The listing builds one solid part. Answer for the finished solid, in the listing's coordinates (mm). Face numbers are marked on the shaded views. Give positions to 0.01 mm unless a question says otherwise; leave off trailing zeros. Write each loop counter-clockwise with the first axis right and the second up, starting at its lowest first coordinate (ties: lowest second). Pieces come first, ordered by that corner, then holes. Notation, with made-up numbers: (55.25, 7.25) - (91.25, 7.25) arc R19 cw to (91.25, 38.25) - close; hole circle Ø3 at (34, -14.5). An arc over 180 degrees is marked (long way). One line per question, with ' | ' between items. Start each with the question number.
1. Find the intervals of material crossed by L1, parallel to X at y = -0.45, z = -81; L2, parallel to X at y = 0.5, z = -32.5; L3, parallel to Z at x = -5, y = 0.4, in increasing order. Write a range as from..to.
2. A cutting plane is placed at C-C (x = -2). Determine the outline of the cut face in (y, z), then the cut area to 4 significant figures.
3. A cutting plane is placed at A-A (z = -71.5). Determine the outline of the cut face in (x, y).
4. The mould has two halves that part along Z. Classify the marked faces 1 and 2: +Z half, -Z half, draft (parallel to the pull), parting line (faces both ways), or undercut.
5. A cutting plane is placed at B-B (y = -1.6). Determine the outline of the cut face in (x, z).
6. A cutting plane is placed at D-D (z = -42). Determine the outline of the cut face in (x, y), then the cut area to 4 significant figures.
7. Given P1, Ø3, axis at x = -39, z = -6.5, coming from the +Y side; P2, Ø3, axis at x = -36.5, y = -2, coming from the -Z side, each flat-ended and moving along its own axis, determine where each tip first touches the part or whether it passes through.
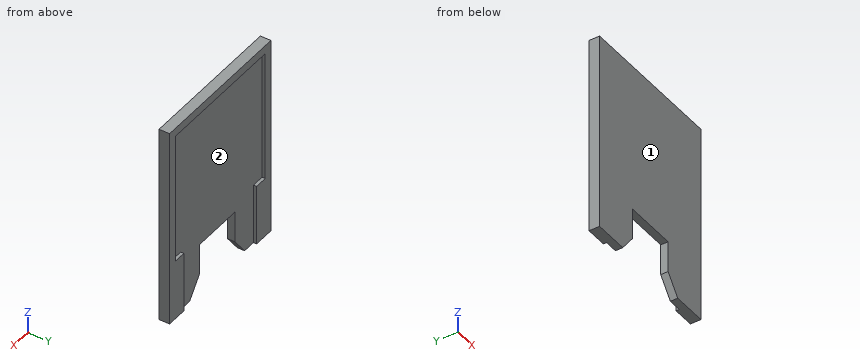
Autodesk Inventor part; units mm, degrees
ref_plane "YZ Plane" through (0, 0, 0) normal (1, 0, 0) x (0, 1, 0)
ref_plane "XZ Plane" through (0, 0, 0) normal (0, 1, 0) x (-1, 0, 0)
ref_plane "XY Plane" through (0, 0, 0) normal (0, 0, 1) x (1, 0, 0)
sketch "Skizze1" plane through (0, 0, 0) normal (0, 1, 0) x (-1, 0, 0)
  line L0 (0, 0) -> (63, 0)
  line L1 (63, 0) -> (63, -63)
  line L2 (63, -63) -> (0, -63)
  line L3 (0, -63) -> (0, 0)
  line L4 (-4, 4) -> (67, 4)
  line L5 (67, 4) -> (67, -92)
  line L6 (67, -92) -> (-4, -92)
  line L7 (-4, -92) -> (-4, 4)
  line L8 (57, -63) -> (6, -63)
  line L9 (6, -63) -> (6, -68)
  line L10 (6, -68) -> (57, -68)
  line L11 (57, -68) -> (57, -63)
  line L12 (44, -68) -> (19, -68)
  line L13 (19, -68) -> (19, -92)
  line L14 (19, -92) -> (44, -92)
  line L15 (44, -92) -> (44, -68)
  line L16 (44, -68) -> (44, -83)
  line L17 (44, -83) -> (44, -93)
  line L18 (44, -93) -> (49.7342, -93)
  line L19 (49.7342, -93) -> (44, -83)
  line L20 (49.1608, -92) -> (44, -92)
  line L21 (19, -83) -> (19, -93)
  line L22 (19, -93) -> (11.5, -93)
  line L23 (11.5, -93) -> (19, -83)
  line L24 (12.25, -92) -> (19, -92)
  line L25 (57, -68) -> (57, -71.1865)
  line L26 (57, -71.1865) -> (57, -92)
  line L27 (6, -68) -> (6, -92)
  point P0 (19, -80)
  dimension "d0" = 63
  dimension "d1" = 63
  dimension "d2" = 71
  dimension "d3" = 96
  dimension "d4" = 51
  dimension "d5" = 5
  dimension "d6" = 6
  dimension "d7" = 6
  dimension "d8" = 4
  dimension "d9" = 25
  dimension "d10" = 24
  dimension "d11" = 15
  dimension "d14" = 10
  dimension "d15" = 10
  dimension "d16" = 15
  dimension "d23" = 13
  dimension "d24" = 13
extrude "Extrusion1" add sketch "Skizze1" along normal blind 1.5 contours L3 L2 L9 L27 L6 L7 L4 L5 L26 L25 L11 L1 L0
sketch "Skizze2" plane through (0, 0, 0) normal (0, -1, 0) x (1, 0, 0)
  line L0 (4, 4) -> (4, -92)
  line L1 (-57, -92) -> (-67, -92)
  line L2 (4, 4) -> (-67, 4)
  line L3 (-67, 4) -> (-67, -92)
  line L4 (-67, -92) -> (4, -92)
  line L5 (4, -92) -> (4, 4)
  line L6 (-19, -92) -> (-44, -92)
  line L7 (-44, -92) -> (-44, -68)
  line L8 (-44, -68) -> (-19, -68)
  line L9 (-19, -68) -> (-19, -92)
  line L10 (-6, -92) -> (-6, -63)
  line L11 (-57, -63) -> (-57, -92)
  line L12 (-44, -68) -> (-44, -83)
  line L13 (-44, -83) -> (-44, -92)
  line L14 (-44, -83) -> (-44, -93)
  line L15 (-44, -83) -> (-34, -83) construction
  line L16 (-44, -93) -> (-51.5, -93)
  line L17 (-51.5, -93) -> (-44, -83)
  line L18 (-19, -83) -> (-19, -93)
  line L19 (-19, -93) -> (-11.5, -93)
  line L20 (-11.5, -93) -> (-19, -83)
  point P0 (0, 0)
  point P1 (-50.75, -92)
  point P2 (-12.25, -92)
  dimension "d19" = 25
  dimension "d20" = 24
  dimension "d21" = 13
  dimension "d22" = 13
  dimension "d25" = 15
  dimension "d26" = 10
  dimension "d27" = 90
  dimension "d28" = 7.5
  dimension "d29" = 7.5
extrude "Extrusion2" add sketch "Skizze2" along normal blind 3.5 contours L0 L4 L20 L9 L8 L7 L17 L1 L3 L2
equation "\"d15\" = d14"
equation "\"Biegeradius\" = Stärke"
equation "\"BreiteBiegungsfreistellung\" = Stärke"
equation "\"TiefeBiegungsfreistellung\" = 0.5 * Stärke"
equation "\"GrößeEckenfreistellung\" = 4 * Stärke"
equation "\"MinimalRest\" = 2 * Stärke"
equation "\"Übergangsradius\" = Biegeradius"
equation "\"JacobiRadiusGröße\" = Biegeradius"
equation "\"Abstandsgröße\" = Stärke"
Determined:
1) L1: -67..-44, -19..4 | L2: -67..-63, 0..4 | L3: -92..-63, 0..4
2) outline: (-3.5, -92) - (1.5, -92) - (1.5, -63) - (0, -63) - (0, 0) - (1.5, 0) - (1.5, 4) - (-3.5, 4) - close | area: 385.5 mm2
3) outline: (-67, -3.5) - (-44, -3.5) - (-44, 0) - (-57, 0) - (-57, 1.5) - (-67, 1.5) - close; (-19, -3.5) - (4, -3.5) - (4, 1.5) - (-6, 1.5) - (-6, 0) - (-19, 0) - close
4) face 1: draft | face 2: undercut
5) outline: (-67, -92) - (-50.75, -92) - (-44, -83) - (-44, -68) - (-19, -68) - (-19, -83) - (-12.25, -92) - (4, -92) - (4, 4) - (-67, 4) - close
6) outline: (-67, -3.5) - (4, -3.5) - (4, 1.5) - (0, 1.5) - (0, 0) - (-63, 0) - (-63, 1.5) - (-67, 1.5) - close | area: 260.5 mm2
7) P1: y = 0 | P2: z = -68
